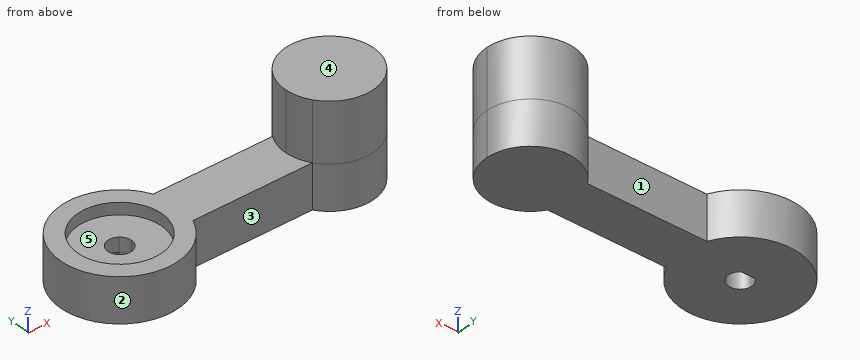
```python
from build123d import *

# Parameters (mm, degrees)
F0_R     = 18.1102
F1_DEPTH = 19.05
F2_DEPTH = 25.4
F3_DEPTH = 5.08
F4_DEPTH = 11.176
F5_DEPTH = 20.32


with BuildPart() as f1:
    # F0 (on Top) → F1 (new body)
    with BuildSketch(Plane.XY):
        with BuildLine():
            ThreePointArc((23.279485, -10.16), (24.86422, -5.189465), (25.4, 0))
            ThreePointArc((25.4, 0), (24.86422, 5.189465), (23.279485, 10.16))
            ThreePointArc((23.279485, 10.16), (-25.4, 0), (23.279485, -10.16))
        make_face()
        Circle(F0_R, mode=Mode.SUBTRACT)
        Circle(F0_R)
        with BuildLine():
            ThreePointArc((3.127605, 4.0513), (4.593601, 2.256939), (5.1181, 0))
            ThreePointArc((5.1181, 0), (-2.256939, -4.593601), (-3.127605, 4.0513))
            ThreePointArc((-3.127605, 4.0513), (0, 5.1181), (3.127605, 4.0513))
        make_face(mode=Mode.SUBTRACT)
        with BuildLine():
            ThreePointArc((-3.127605, 4.0513), (-2.256939, -4.593601), (5.1181, 0))
            ThreePointArc((5.1181, 0), (4.593601, 2.256939), (3.127605, 4.0513))
            Line((3.127605, 4.0513), (-3.127605, 4.0513))
        make_face()
        with BuildLine():
            Line((-3.127605, 4.0513), (3.127605, 4.0513))
            ThreePointArc((3.127605, 4.0513), (0, 5.1181), (-3.127605, 4.0513))
        make_face()
        with BuildLine():
            Line((72.39, 0), (25.4, 0))
            ThreePointArc((25.4, 0), (24.86422, -5.189465), (23.279485, -10.16))
            Line((23.279485, -10.16), (75.325507, -10.16))
            ThreePointArc((75.325507, -10.16), (73.138585, -5.287788), (72.39, 0))
        make_face()
        with BuildLine():
            ThreePointArc((23.279485, 10.16), (24.86422, 5.189465), (25.4, 0))
            Line((25.4, 0), (72.39, 0))
            ThreePointArc((72.39, 0), (73.138585, 5.287788), (75.325507, 10.16))
            Line((75.325507, 10.16), (23.279485, 10.16))
        make_face()
        with BuildLine():
            ThreePointArc((75.325507, 10.16), (73.138585, 5.287788), (72.39, 0))
            ThreePointArc((72.39, 0), (73.138585, -5.287788), (75.325507, -10.16))
            ThreePointArc((75.325507, -10.16), (96.727788, -18.301415), (110.49, 0))
            ThreePointArc((110.49, 0), (96.727788, 18.301415), (75.325507, 10.16))
        make_face()
    extrude(amount=-F1_DEPTH)

    # F0 (on Top) → F2 (join)
    with BuildSketch(Plane.XY):
        with BuildLine():
            ThreePointArc((75.325507, 10.16), (73.138585, 5.287788), (72.39, 0))
            ThreePointArc((72.39, 0), (73.138585, -5.287788), (75.325507, -10.16))
            ThreePointArc((75.325507, -10.16), (96.727788, -18.301415), (110.49, 0))
            ThreePointArc((110.49, 0), (96.727788, 18.301415), (75.325507, 10.16))
        make_face()
    extrude(amount=F2_DEPTH)

    # F0 (on Top) → F3 (cut)
    with BuildSketch(Plane.XY):
        Circle(F0_R)
        with BuildLine():
            ThreePointArc((3.127605, 4.0513), (4.593601, 2.256939), (5.1181, 0))
            ThreePointArc((5.1181, 0), (-2.256939, -4.593601), (-3.127605, 4.0513))
            ThreePointArc((-3.127605, 4.0513), (0, 5.1181), (3.127605, 4.0513))
        make_face(mode=Mode.SUBTRACT)
        with BuildLine():
            ThreePointArc((-3.127605, 4.0513), (-2.256939, -4.593601), (5.1181, 0))
            ThreePointArc((5.1181, 0), (4.593601, 2.256939), (3.127605, 4.0513))
            Line((3.127605, 4.0513), (-3.127605, 4.0513))
        make_face()
        with BuildLine():
            Line((-3.127605, 4.0513), (3.127605, 4.0513))
            ThreePointArc((3.127605, 4.0513), (0, 5.1181), (-3.127605, 4.0513))
        make_face()
    extrude(amount=-F3_DEPTH, mode=Mode.SUBTRACT)

    # F0 (on Top) → F4 (cut)
    with BuildSketch(Plane.XY):
        with BuildLine():
            ThreePointArc((-3.127605, 4.0513), (-2.256939, -4.593601), (5.1181, 0))
            ThreePointArc((5.1181, 0), (4.593601, 2.256939), (3.127605, 4.0513))
            Line((3.127605, 4.0513), (-3.127605, 4.0513))
        make_face()
        with BuildLine():
            Line((-3.127605, 4.0513), (3.127605, 4.0513))
            ThreePointArc((3.127605, 4.0513), (0, 5.1181), (-3.127605, 4.0513))
        make_face()
    extrude(amount=-F4_DEPTH, mode=Mode.SUBTRACT)

    # F0 (on Top) → F5 (cut)
    with BuildSketch(Plane.XY):
        with BuildLine():
            ThreePointArc((-3.127605, 4.0513), (-2.256939, -4.593601), (5.1181, 0))
            ThreePointArc((5.1181, 0), (4.593601, 2.256939), (3.127605, 4.0513))
            Line((3.127605, 4.0513), (-3.127605, 4.0513))
        make_face()
    extrude(amount=-F5_DEPTH, mode=Mode.SUBTRACT)


solid = f1.part
```
CAD build for the part. Positions are in the model's coordinates, mm. Face numbers are marked on the shaded views. A direction names the side the tool comes from. Coordinates: 2 decimals unless noted, no trailing zeros. Order: outer loops, then holes, each group sorted by start corner. A loop starts at its lowest first (then second) coordinate and runs counter-clockwise, first axis right, second up.
(1) Saw through at C-C, the plane z = -15. Write the cut outline in (x, y).
Solution:
outline: (23.28, -10.16) - (75.33, -10.16) arc R19.05 ccw (long way) to (75.33, 10.16) - (23.28, 10.16) arc R25.4 ccw (long way) to start; hole (-3.13, 4.05) arc R5.12 ccw (long way) to (5.12, 0) arc R5.12 ccw to (3.13, 4.05) - close
(2) Drill centre lines: L1, parallel to Y at x = 0, z = -8.25; L2, parallel to Y at x = 0, z = -17; L3, parallel to Z at x = 50, y = 4.5. Where is each one in solid material? Low to high.
Solution:
L1: y = -25.4 to -5.12, 5.12 to 25.4
L2: y = -25.4 to -5.12, 4.05 to 25.4
L3: z = -19.05 to 0
(3) Saw through at B-B, the plane y = 12.5. Write the cut outline in (x, z), and give its area (3 significant figures).
Solution:
outline: (-22.11, -19.05) - (22.11, -19.05) - (22.11, 0) - (13.1, 0) - (13.1, -5.08) - (-13.1, -5.08) - (-13.1, 0) - (-22.11, 0) - close; (77.06, -19.05) - (105.82, -19.05) - (105.82, 25.4) - (77.06, 25.4) - close
area: 1,990 mm2
(4) Saw through at A-A, the plane x = 0. Write the cut outline in (y, z), and give its area (3 significant figures).
Solution:
outline: (-25.4, -19.05) - (-5.12, -19.05) - (-5.12, -5.08) - (-18.11, -5.08) - (-18.11, 0) - (-25.4, 0) - close; (4.05, -19.05) - (25.4, -19.05) - (25.4, 0) - (18.11, 0) - (18.11, -5.08) - (5.12, -5.08) - (5.12, -11.18) - (4.05, -11.18) - close
area: 649 mm2
(5) Saw through at D-D, the plane y = -3.5. Write the cut outline in (x, z), and give its area (3 significant figures).
Solution:
outline: (-25.16, -19.05) - (-3.73, -19.05) - (-3.73, -5.08) - (-17.77, -5.08) - (-17.77, 0) - (-25.16, 0) - close; (3.73, -19.05) - (110.17, -19.05) - (110.17, 25.4) - (72.71, 25.4) - (72.71, 0) - (17.77, 0) - (17.77, -5.08) - (3.73, -5.08) - close
area: 3,240 mm2
(6) Pin check, flat tips, straight feed: pin 1 Ø2 at (x, z) = (57, -7) entering from +Y; pin 2 Ø10 at (x, z) = (7, 2.5) entering from +Y; pin 3 Ø18 at (x, y) = (-3, 0.5) entering from +Z; pin 4 Ø10 at (x, z) = (40, 9) entering from -Y. Stop position of each tip, or through.
Solution:
pin 1: stops at y = 10.16
pin 2: stops at y = 25.26
pin 3: stops at z = -5.08
pin 4: passes through
(7) Which spindle directions (+Z, -Z, +X, -X, +Y, -Y) get a long thin tool onto all of the face, cutting with end or side? Do the marked faces 1, 2 and 3. Say none if no direction does.
Solution:
face 1: +Z, -Z, +Y
face 2: +Z, -Z
face 3: +Z, -Z, -Y
(8) Mould opens along X. For the marked faces 4 and 5 say: released by +X, released by -X, zero draft, split by the parting line, or undercut.
Solution:
face 4: zero draft
face 5: undercut
